For this review, take the finished solid that the model builds, in its own axes (mm). Face numbers are marked on the shaded views. A direction names the side the tool comes from. Give positions to 0.01 mm unless a question says otherwise; leave off trailing zeros. Write each loop counter-clockwise with the first axis right and the second up, starting at its lowest first coordinate (ties: lowest second). Pieces come first, ordered by that corner, then holes. Notation, with made-up numbers: (39.5, 51.5) -> (71.5, 51.5) arc R28 ccw to (71.5, 80.5) -> close; hole circle Ø1 at (1, -17.5). An arc over 180 degrees is marked (long way). Return JSON: item names as keys, results as strings.
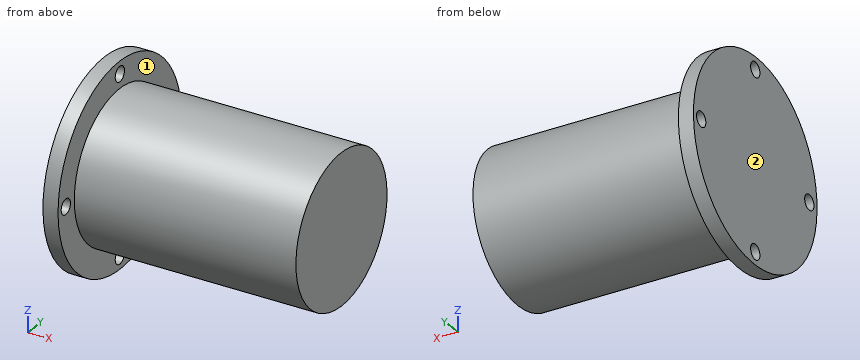
from build123d import *

# Parameters (mm, degrees)
SKETCH1_R           = 14.75
BOSS_EXTRUDE1_DEPTH = 47
SKETCH2_R           = 20
SKETCH2_R_2         = 1.5
BOSS_EXTRUDE2_DEPTH = 3


with BuildPart() as part:
    # Sketch1 → Boss-Extrude1 (new body)
    with BuildSketch(Plane(origin=(0, 0, 0), x_dir=(0, 0, -1), z_dir=(1, 0, 0))):
        Circle(SKETCH1_R)
    extrude(amount=BOSS_EXTRUDE1_DEPTH)

    # Sketch2 → Boss-Extrude2 (add)
    with BuildSketch(Plane.ZY):
        Circle(SKETCH2_R)
        with Locations((0, 17.5)):
            Circle(SKETCH2_R_2, mode=Mode.SUBTRACT)
        with Locations((17.5, 0)):
            Circle(SKETCH2_R_2, mode=Mode.SUBTRACT)
        with Locations((0, -17.5)):
            Circle(SKETCH2_R_2, mode=Mode.SUBTRACT)
        with Locations((-17.5, 0)):
            Circle(SKETCH2_R_2, mode=Mode.SUBTRACT)
    extrude(amount=-BOSS_EXTRUDE2_DEPTH)


solid = part.part
1. Add section A-A, the plane z = 0. State the section outline as (x, y) points.
Results found:
{"outline": "(0, -20) -> (3, -20) -> (3, -19) -> (0, -19) -> close; (0, -16) -> (3, -16) -> (3, -14.75) -> (47, -14.75) -> (47, 14.75) -> (3, 14.75) -> (3, 16) -> (0, 16) -> close; (0, 19) -> (3, 19) -> (3, 20) -> (0, 20) -> close"}
2. Add section D-D, the plane x = 11. State the section outline as (y, z) points.
Results found:
{"outline": "circle Ø29.5 at (0, 0)"}
3. For pin 1 (12 mm diameter, centred on x = 25.5, y = 3.5, fed in from -Z); pin 2 (3.5 mm diameter, centred on y = 17.5, z = 0, fed in from +X); pin 3 (5 mm diameter, centred on x = 25.5, y = -6.5, fed in from -Z), all flat-tipped, find the tip position at first contact; note any pin that passes through.
Results found:
{"pin 1": "stops at z = -14.75", "pin 2": "stops at x = 3", "pin 3": "stops at z = -14.2"}
4. Add section B-B, the plane y = -17.5. State the section outline as (x, z) points.
Results found:
{"outline": "(0, -9.68) -> (3, -9.68) -> (3, -1.5) -> (0, -1.5) -> close; (0, 1.5) -> (3, 1.5) -> (3, 9.68) -> (0, 9.68) -> close"}
5. To check wall thickness, follow probe 1 along Y at (x, z) = (1, 0); probe 2 along X at (y, z) = (18, -1.5); probe 3 along Y at (x, z) = (1.6, 17.5). State the ranges of each line that lie inside material, in increasing order.
Results found:
{"probe 1": "y = -20 to -19, -16 to 16, 19 to 20", "probe 2": "x = 0 to 3", "probe 3": "y = -9.68 to -1.5, 1.5 to 9.68"}
6. For the marked faces 1 and 2, list the 3-axis set-ups (+Z, -Z, +X, -X, +Y, -Y) from which the entire face can be reached by the end or side of a thin tool; tool diameter is ignored.
Results found:
{"face 1": "+X", "face 2": "+Z, -Z, -X, +Y, -Y"}
